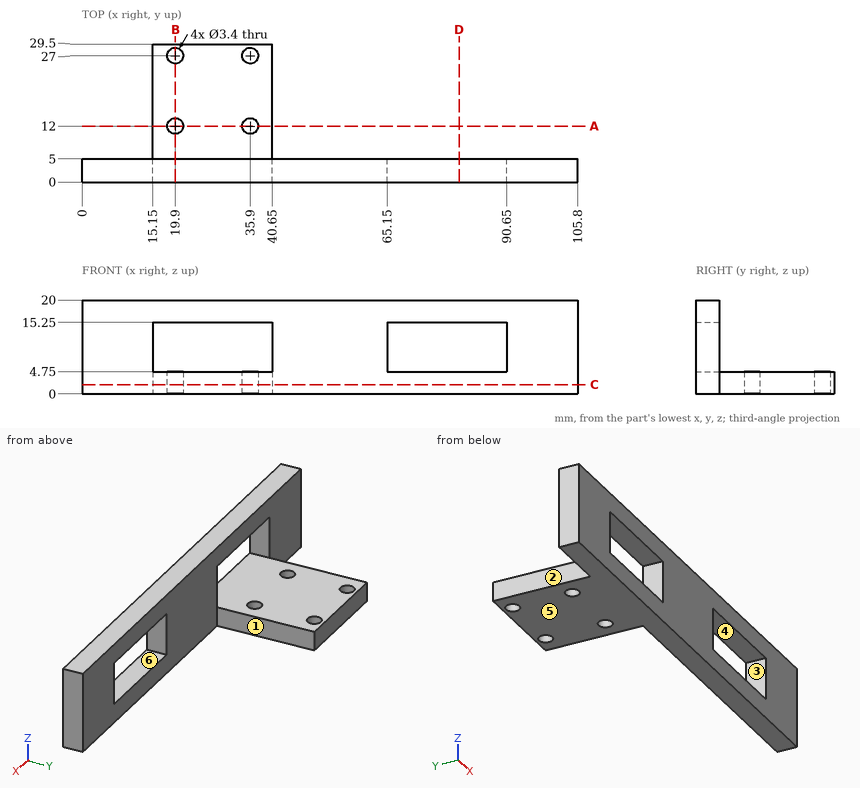
Here's the drawing with two shaded views (mm, measured from the low corner). I have some questions. A direction names the side the tool comes from. Round coordinates to 2 decimals unless told otherwise and drop trailing zeros. Loops run counter-clockwise (first coordinate to the right, second up) from the corner with the lowest first, then second, coordinate; pieces in that order, holes last. Notation, with made-up numbers: (84, 66) - (113, 66) arc R24 cw to (113, 92) - close; hole circle Ø4 at (29, 37.5). An arc over 180 degrees is marked (long way). Use CSV: the item, a comma, the result in double quotes. Start each with the question number.
1) For pin 1 Ø5 at (x, z) = (51, 3) entering from -Y; pin 2 Ø6 at (x, z) = (46, 7) entering from +Y; pin 3 Ø10 at (y, z) = (15, 6) entering from +X; pin 4 Ø5 at (y, z) = (19.5, 3) entering from -X, each with a flat end and sliding along its axis, tell me the tip position at first contact or that it passes through.
2) If we section it at B-B on x = 19.9: Write out the boundary of the cut face in (y, z), plus the area to 3 significant figures.
3) For the marked faces 5 and 6, which set-ups out of +Z, -Z, +X, -X, +Y, -Y let a thin tool reach every point of the face, with its end or its side?
4) We'd pull the mould along X, two halves only. Please class the marked faces 1, 2, 3 and 4: released by +X, released by -X, zero draft, split by the parting line, or undercut.
5) If we section it at D-D on x = 80.5: Write out the boundary of the cut face in (y, z), plus the area to 3 significant figures.
6) Please list where these lines run through material, in increasing order: probe 1 along X at (y, z) = (1.75, 12.25); probe 2 along Y at (x, z) = (19.9, 3.6); probe 3 along Z at (x, y) = (24, 24.5). Write a range as [from, to].
7) If we section it at C-C on z = 2: Write out the boundary of the cut face in (x, y).
8) If we section it at A-A on y = 12: Write out the boundary of the cut face in (x, z), plus the area to 3 significant figures.
Geometry results:
1,pin 1,"stops at y = 0"
1,pin 2,"stops at y = 5"
1,pin 3,"stops at x = 40.65"
1,pin 4,"stops at x = 15.15"
2,outline,"(0, 0) - (10.3, 0) - (10.3, 4.75) - (0, 4.75) - close; (0, 15.25) - (5, 15.25) - (5, 20) - (0, 20) - close; (13.7, 0) - (25.3, 0) - (25.3, 4.75) - (13.7, 4.75) - close; (28.7, 0) - (29.5, 0) - (29.5, 4.75) - (28.7, 4.75) - close"
2,area,"132 mm2"
3,face 5,"-Z, +X, -X, +Y, -Y"
3,face 6,"+Y, -Y"
4,face 1,"released by +X"
4,face 2,"released by -X"
4,face 3,"undercut"
4,face 4,"undercut"
5,outline,"(0, 0) - (5, 0) - (5, 4.75) - (0, 4.75) - close; (0, 15.25) - (5, 15.25) - (5, 20) - (0, 20) - close"
5,area,"47.5 mm2"
6,probe 1,"x = [0, 15.15], [40.65, 65.15], [90.65, 105.8]"
6,probe 2,"y = [0, 10.3], [13.7, 25.3], [28.7, 29.5]"
6,probe 3,"z = [0, 4.75]"
7,outline,"(0, 0) - (105.8, 0) - (105.8, 5) - (40.65, 5) - (40.65, 29.5) - (15.15, 29.5) - (15.15, 5) - (0, 5) - close; hole circle Ø3.4 at (19.9, 12); hole circle Ø3.4 at (19.9, 27); hole circle Ø3.4 at (35.9, 12); hole circle Ø3.4 at (35.9, 27)"
8,outline,"(15.15, 0) - (18.2, 0) - (18.2, 4.75) - (15.15, 4.75) - close; (21.6, 0) - (34.2, 0) - (34.2, 4.75) - (21.6, 4.75) - close; (37.6, 0) - (40.65, 0) - (40.65, 4.75) - (37.6, 4.75) - close"
8,area,"88.8 mm2"
